The drawing under review shows one solid part. Ordinate dimensions are in mm from its lowest x, y, z. Coordinates: 2 decimals unless noted, no trailing zeros. Loops run counter-clockwise (first coordinate to the right, second up) from the corner with the lowest first, then second, coordinate; pieces in that order, holes last. Notation, with made-up numbers: (71.25, -11.5) - (87.25, -11.5) arc R19 ccw to (87.25, 11.5) - close; hole circle Ø8 at (-38.5, -19). An arc over 180 degrees is marked (long way). Use one line per item in the form item = value. Start each with the question number.
1. Add section C-C on z = 51. Give the boundary of the cut face in (x, y), and give its area (3 significant figures).
2. To check wall thickness, follow probe 1 along Y at (x, z) = (18, 18); probe 2 along Z at (x, y) = (11, 27.5); probe 3 along Y at (x, z) = (4, 18). State the ranges of each line that lie inside material, in increasing order.
3. Draft analysis for pull direction Z (two halves, no side actions). For the marked faces 1, 2 and 3, state which applies: +Z half, -Z half, draft (parallel to the pull), parting line (faces both ways), or undercut.
4. Add section B-B on x = 18. Give the boundary of the cut face in (y, z), and give its area (3 significant figures).
5. For pin 1 Ø10 at (y, z) = (9.5, 15.5) entering from +X; pin 2 Ø0.9 at (x, y) = (17.5, 4) entering from -Z; pin 3 Ø12 at (x, y) = (5, 25) entering from -Z, all flat-tipped, find the tip position at first contact; note any pin that passes through.
6. Add section A-A on z = 18. Give the boundary of the cut face in (x, y).
7. Add section D-D on y = 4. Give the boundary of the cut face in (x, z), and give its area (3 significant figures).
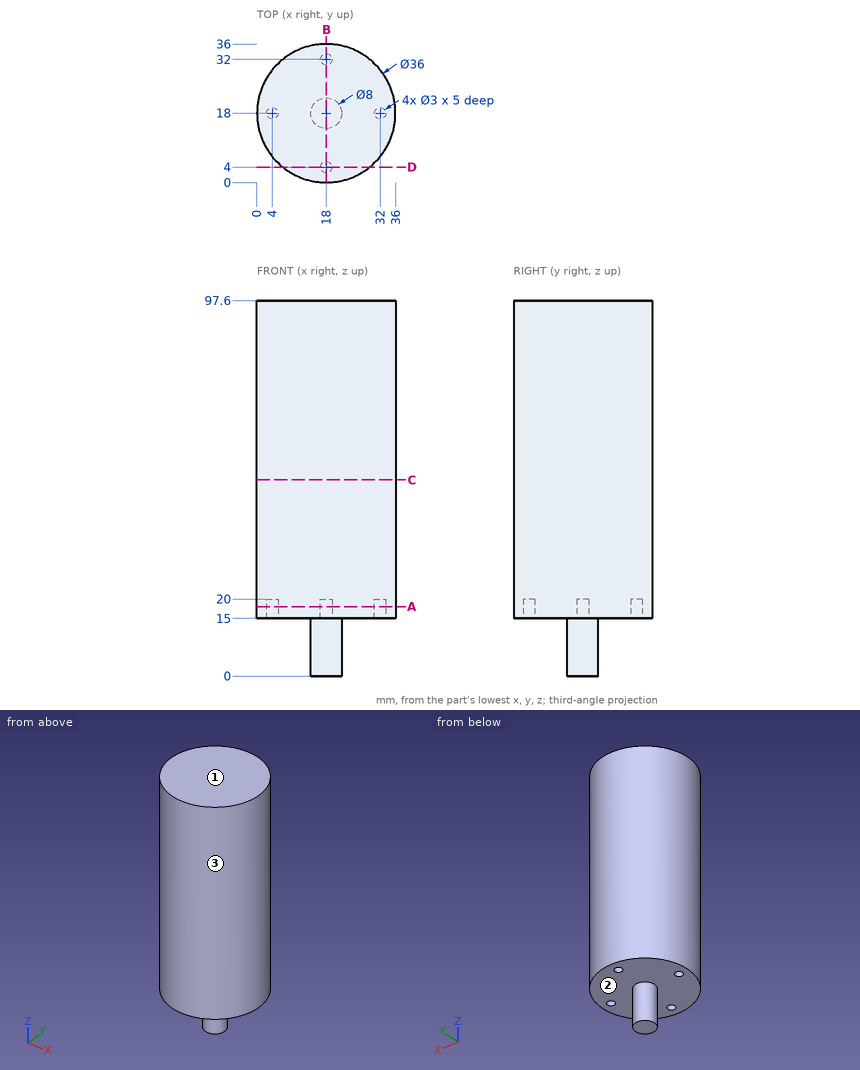
Conclusion:
q1.outline = circle Ø36 at (18, 18)
q1.area = 1,020 mm^2
q2.probe_1 = 0 to 2.5, 5.5 to 30.5, 33.5 to 36
q2.probe_2 = 15 to 97.6
q2.probe_3 = 6.69 to 16.5, 19.5 to 29.31
q3.face_1 = +Z half
q3.face_2 = -Z half
q3.face_3 = draft
q4.outline = (0, 15) - (2.5, 15) - (2.5, 20) - (5.5, 20) - (5.5, 15) - (14, 15) - (14, 0) - (22, 0) - (22, 15) - (30.5, 15) - (30.5, 20) - (33.5, 20) - (33.5, 15) - (36, 15) - (36, 97.6) - (0, 97.6) - close
q4.area = 3,060 mm^2
q5.pin_1 = 35.66
q5.pin_2 = 20
q5.pin_3 = 15
q6.outline = circle Ø36 at (18, 18); hole circle Ø3 at (4, 18); hole circle Ø3 at (18, 4); hole circle Ø3 at (18, 32); hole circle Ø3 at (32, 18)
q7.outline = (6.69, 15) - (16.5, 15) - (16.5, 20) - (19.5, 20) - (19.5, 15) - (29.31, 15) - (29.31, 97.6) - (6.69, 97.6) - close
q7.area = 1,850 mm^2
